Read the model definition and answer for the solid it produces. Units are mm, in the model's axes. Face numbers are marked on the shaded views. A direction names the side the tool comes from. Round coordinates to 2 decimals unless told otherwise and drop trailing zeros. Write each loop counter-clockwise with the first axis right and the second up, starting at its lowest first coordinate (ties: lowest second). Pieces come first, ordered by that corner, then holes. Notation, with made-up numbers: (66.5, 36.25) - (89.5, 36.25) arc R31 ccw to (89.5, 71.25) - close; hole circle Ø7 at (87, 32.5). An arc over 180 degrees is marked (long way). Use one line per item in the form item = value. Start each with the question number.
1) Consider line 1 along Z through (x, y) = (12.5, -48.1); line 2 along Y through (x, z) = (7.5, 4.1); line 3 along Y through (x, z) = (6, 5.3). Determine where each line is inside the solid, lowest interval first. Write a range as from..to.
2) The part is cut by section B-B, the plane x = 12.5. Give the vertices of the cut face in (y, z).
3) Each of these flat-tipped pins is pushed along its axis until it touches: pin 1 (0.5 mm diameter, centred on x = 5.5, z = 5.5, fed in from +Y); pin 2 (1 mm diameter, centred on x = 13, z = 2, fed in from -Y); pin 3 (1 mm diameter, centred on x = 4.5, y = -33, fed in from +Z); pin 4 (4 mm diameter, centred on x = 7.5, y = 5, fed in from +Z). Where does it stop, or does it pass through?
4) The part is cut by section A-A, the plane z = 2.5. Give the vertices of the cut face in (x, y).
5) The part is cut by section D-D, the plane x = 8. Give the vertices of the cut face in (y, z), plus the area to 3 significant figures.
6) The part is cut by section C-C, the plane y = -9. Give the vertices of the cut face in (x, z).
7) For the marked faces 1 and 2, determine the directions among +Z, -Z, +X, -X, +Y, -Y from which every point of the face is accessible in a straight line to the end or side of a thin tool.
from build123d import *

# Parameters (mm, degrees)
BOSS_EXTRUDE1_DEPTH = 5
SKETCH2_W           = 10
SKETCH2_H           = 10
BOSS_EXTRUDE2_DEPTH = 5.93
FILLET1_R           = 1
SKETCH3_R           = 1.029396526
CUT_EXTRUDE1_DEPTH  = 0.5


with BuildPart() as part:
    # Sketch1 → Boss-Extrude1 (new body)
    with BuildSketch(Plane.XY):
        Polygon((10, 12), (10, -15.48), (0, -15.48), (0, -48.42), (15, -48.42), (15, 12), align=None)
    extrude(amount=BOSS_EXTRUDE1_DEPTH)

    # Sketch2 → Boss-Extrude2 (add)
    with BuildSketch(Plane(origin=(0, 0, 0), x_dir=(-1, 0, 0), z_dir=(0, 0, -1))):
        with Locations((-5, -43.42)):
            Rectangle(SKETCH2_W, SKETCH2_H)
    extrude(amount=-BOSS_EXTRUDE2_DEPTH)

    # Fillet1
    fillet1_edges = [part.edges().sort_by_distance(p)[0] for p in [
        (10, 12, 2.5),
        (15, 12, 2.5),
        (12.5, 12, 5),
    ]]
    fillet(fillet1_edges, radius=FILLET1_R)

    # Sketch3 → Cut-Extrude1 (cut)
    with BuildSketch(Plane.XZ.offset(48.42)):
        with Locations((12.5, 2.5)):
            Circle(SKETCH3_R)
    extrude(amount=-CUT_EXTRUDE1_DEPTH, mode=Mode.SUBTRACT)


solid = part.part
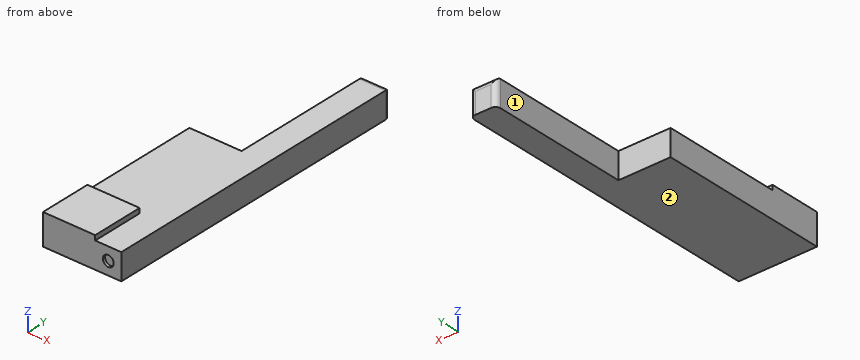
Geometry results:
q1.line_1 = 0..1.47, 3.53..5
q1.line_2 = -48.42..-15.48
q1.line_3 = -48.42..-38.42
q2.outline = (-48.42, 0) - (12, 0) - (12, 4) arc R1 ccw to (11, 5) - (-48.42, 5) - (-48.42, 3.53) - (-47.92, 3.53) - (-47.92, 1.47) - (-48.42, 1.47) - close
q3.pin_1 = -38.42
q3.pin_2 = -48.42
q3.pin_3 = 5
q3.pin_4 = through
q4.outline = (0, -48.42) - (11.47, -48.42) - (11.47, -47.92) - (13.53, -47.92) - (13.53, -48.42) - (15, -48.42) - (15, 11) arc R1 ccw to (14, 12) - (11, 12) arc R1 ccw to (10, 11) - (10, -15.48) - (0, -15.48) - close
q5.outline = (-48.42, 0) - (-15.48, 0) - (-15.48, 5) - (-38.42, 5) - (-38.42, 5.93) - (-48.42, 5.93) - close
q5.area = 174 mm2
q6.outline = (10, 0) - (15, 0) - (15, 5) - (10, 5) - close
q7.face_1 = +Z, -Z, -X, +Y
q7.face_2 = -Z, +X, -X, +Y, -Y
